```python
from build123d import *

# Parameters (mm, degrees)
CHAMFER1_SIZE           = 0.635
FILLET3_R               = 0.508
CUT_EXTRUDE8_REACH      = 49.123
CIRPATTERN1_COUNT       = 6
FILLET4_R               = 0.762
CUT_EXTRUDE9_DEPTH      = 41.411152568
CUT_EXTRUDE9_DEPTH_BACK = 41.411152568
SKETCH15_W              = 0.254
SKETCH15_H              = 25.164906623
CHAMFER2_SIZE           = 0.762


with BuildPart() as part:
    # Sketch1 → mainBody (revolve)
    with BuildSketch(Plane(origin=(0, 0, 0), x_dir=(0, 0, -1), z_dir=(1, 0, 0)), mode=Mode.PRIVATE) as mainbody_sk:
        Polygon((-6.096, 38.1), (-6.096, 8.705990249), (0, 0), (0, -7.057106074), (-1.905, -7.057106074), (-1.905, -0.707106074), (-7.9375, -0.707106074), (-7.9375, 5.642893926), (-9.525, 5.642893926), (-9.525, 38.1), align=None)
    revolve(mainbody_sk.sketch.rotate(Axis((0, 0, 0), (0, 1, 0)), 180), axis=Axis((0, 0, 0), (0, 1, 0)))

    # Chamfer1
    chamfer1_edges = [part.edges().sort_by_distance(p)[0] for p in [
        (0, 38.1, 6.096),
    ]]
    chamfer(chamfer1_edges, length=CHAMFER1_SIZE)

    # Fillet3
    fillet3_edges = [part.edges().sort_by_distance(p)[0] for p in [
        (0, 38.1, 9.525),
    ]]
    fillet(fillet3_edges, radius=FILLET3_R)

    # Cut-Extrude8: up to this cone (the profile starts inside it)
    cut_extrude8_end = Plane(origin=(0, 38.1, 0), z_dir=(0, 1, 0)).offset(-38.099999) * Cone(1e-06, 80.104377604, 114.400906206, align=(Align.CENTER, Align.CENTER, Align.MIN), mode=Mode.PRIVATE)
    # Sketch13 → Cut-Extrude8 (cut, up to the surface)
    with BuildSketch(Plane(origin=(0, 38.1, 0), x_dir=(1, 0, 0), z_dir=(0, 1, 0)), mode=Mode.PRIVATE) as cut_extrude8_sk1:
        Polygon((-1.27, 8.001), (1.27, 8.001), (2.27589157, 2.296305428), (-2.27589157, 2.296305428), align=None)
    cut_extrude8_tool1 = extrude(cut_extrude8_sk1.sketch, amount=-CUT_EXTRUDE8_REACH, mode=Mode.PRIVATE) & cut_extrude8_end
    cut_extrude8 = cut_extrude8_tool1.solids().sort_by_distance((0, 38.1, -4.878937))[0]
    add(cut_extrude8, mode=Mode.SUBTRACT)

    # CirPattern1: Cut-Extrude8 ×6 about axis
    cirpattern1_axis = Axis((0, 0, 0), (0, 1, 0))
    for i in range(1, CIRPATTERN1_COUNT):
        add(cut_extrude8.rotate(cirpattern1_axis, i * 360 / CIRPATTERN1_COUNT), mode=Mode.SUBTRACT)

    # Fillet4
    fillet4_edges = [part.edges().sort_by_distance(p)[0] for p in [
        (0, -0.707106074, 1.905),
    ]]
    fillet(fillet4_edges, radius=FILLET4_R)

    # Sketch15 → Cut-Extrude9 (cut, two sides: drawn at the far end of the back side and taken through both)
    with BuildSketch(Plane.XY.offset(-CUT_EXTRUDE9_DEPTH_BACK)):
        with Locations((0, -13.289559386)):
            Rectangle(SKETCH15_W, SKETCH15_H)
    extrude(amount=CUT_EXTRUDE9_DEPTH + CUT_EXTRUDE9_DEPTH_BACK, mode=Mode.SUBTRACT)

    # Chamfer2
    chamfer2_edges = [part.edges().sort_by_distance(p)[0] for p in [
        (0, -0.707106074, 7.9375),
    ]]
    chamfer(chamfer2_edges, length=CHAMFER2_SIZE)


solid = part.part
```
Source: CAD feature listing. Evaluate the final solid. Frame: model axes, mm. A direction names the side the tool comes from. Coordinates: 2 decimals unless noted, no trailing zeros. Loops run counter-clockwise (first coordinate to the right, second up) from the corner with the lowest first, then second, coordinate; pieces in that order, holes last. Notation, with made-up numbers: M 36,74.25 L 52,74.25 A25 cw 52,98.25 Z; hole C 9.25,-27 d2. An arc over 180 degrees is marked long. Put each result on its own line as item: value. Start each with the question number.
1) Ray query, L1, parallel to Z at x = 6.5, y = 36.5; L2, parallel to X at y = 9, z = 0.25; L3, parallel to Y at x = -7, z = -1. Return the intervals inside material, ascending. Write a range as from..to.
2) Pull-direction query (X, two-part tool) for faces 4 (the face through (-1.46, 23.61, -6.92)), 5 (the face through (-1, -7.057, 0)), 6 (the face through (9.3, 21.84, 2.06)); classes: pulls with the +X half, pulls with the -X half, needs draft (parallel to the pull), parting line crosses it, or undercut.
3) Reachability of faces 1 (the face through (0.127, -4, 0)), 2 (the face through (-7, 38.1, 1)), 3 (the face through (-1.455, 23.609, 6.95)) from +Z, -Z, +X, -X, +Y, -Y: full face, straight path, thin tool, end or side. Return the list, or none.
4) Cut plane B-B on y = 3. Return the cut outline in (x, z) (1 decimal).
5) Contact query for flat-ended pins moving along their axis: pin 1 Ø6 at (x, y) = (3, -1) entering from +Z; pin 2 Ø2 at (x, z) = (-5, -2.5) entering from -Y; pin 3 Ø1 at (x, y) = (5, -1) entering from -Z. Output: stop coordinate, or through.
The answers:
1. L1: z = -6.96..-4.74, -2.01..2.01, 4.74..6.96
1. L2: x = -9.52..-6.09, 6.09..9.52
1. L3: y = -0.71..38.1
2. face 4: undercut
2. face 5: needs draft
2. face 6: parting line crosses it
3. face 1: +Z, -Z, -Y
3. face 2: +Z, -Z, +X, -X, +Y
3. face 3: +Y
4. outline: C 0,0 d15.9; hole C 0,0 d4.2
5. pin 1: stops at z = 7.94
5. pin 2: stops at y = -0.71
5. pin 3: stops at z = -5.56
